Check sheet for the modelled part. Datum: model origin and axes. Units: mm. Round coordinates to 2 decimals unless told otherwise and drop trailing zeros. Order: outer loops, then holes, each group sorted by start corner. A loop starts at its lowest first (then second) coordinate and runs counter-clockwise, first axis right, second up. Notation, with made-up numbers: (-15.5, 37) -> (35.5, 37) arc R26 ccw to (35.5, 68) -> close; hole circle Ø1 at (63.25, 41). An arc over 180 degrees is marked (long way). Use CSV: the item, a comma, the result in double quotes.
```python
from build123d import *

# Parameters (mm, degrees)
SKETCH_1_R      = 1.5
EXTRUDE_1_DEPTH = 10


with BuildPart() as part:
    # 草图1 → 凸台-拉伸1 (new body)
    # profile 1 of 7: a face of its own
    with BuildSketch(Plane.XY):
        with BuildLine():
            Line((-33.5, 22.75), (-39.5, 22.75))
            Line((-39.5, 22.75), (-39.5, 9.98))
            Line((-39.5, 9.98), (-39.5, -22.75))
            Line((-39.5, -22.75), (-33.5, -22.75))
            Line((-33.5, -22.75), (39.5, -22.75))
            Line((39.5, -22.75), (39.5, 22.75))
            Line((39.5, 22.75), (6, 22.75))
            Line((6, 22.75), (6, 16.75))
            Line((6, 16.75), (3.578873161, 16.75))
            ThreePointArc((3.578873161, 16.75), (2.780687719, 16.52), (1.982502277, 16.75))
            Line((1.982502277, 16.75), (0, 16.75))
            Line((0, 16.75), (-1.982502277, 16.75))
            ThreePointArc((-1.982502277, 16.75), (-2.780687719, 16.52), (-3.578873161, 16.75))
            Line((-3.578873161, 16.75), (-6, 16.75))
            Line((-6, 16.75), (-6, 22.75))
            Line((-6, 22.75), (-33.5, 22.75))
        make_face()
        with Locations((-36.5, -17.48)):
            Circle(SKETCH_1_R, mode=Mode.SUBTRACT)
        with BuildLine():
            ThreePointArc((-29, -17.48), (-30.5, -18.98), (-32, -17.48))
            ThreePointArc((-32, -17.48), (-30.5, -15.98), (-29, -17.48))
        make_face(mode=Mode.SUBTRACT)
        with Locations((30.5, -17.48)):
            Circle(SKETCH_1_R, mode=Mode.SUBTRACT)
        with Locations((36.5, -17.48)):
            Circle(SKETCH_1_R, mode=Mode.SUBTRACT)
        with Locations((-36.5, 8.02)):
            Circle(SKETCH_1_R, mode=Mode.SUBTRACT)
        with BuildLine():
            ThreePointArc((-29, 8.02), (-30.5, 6.52), (-32, 8.02))
            ThreePointArc((-32, 8.02), (-30.5, 9.52), (-29, 8.02))
        make_face(mode=Mode.SUBTRACT)
        with Locations((-36.5, 18.02)):
            Circle(SKETCH_1_R, mode=Mode.SUBTRACT)
        with Locations((30.5, 8.02)):
            Circle(SKETCH_1_R, mode=Mode.SUBTRACT)
        with Locations((36.5, 8.02)):
            Circle(SKETCH_1_R, mode=Mode.SUBTRACT)
        with Locations((36.5, 18.02)):
            Circle(SKETCH_1_R, mode=Mode.SUBTRACT)
    # profile 2 of 7: a face of its own
    with BuildSketch(Plane.XY):
        with BuildLine():
            Line((-33.5, 22.75), (-39.5, 22.75))
            Line((-39.5, 22.75), (-39.5, 9.98))
            Line((-39.5, 9.98), (-39.5, -22.75))
            Line((-39.5, -22.75), (-33.5, -22.75))
            Line((-33.5, -22.75), (39.5, -22.75))
            Line((39.5, -22.75), (39.5, 22.75))
            Line((39.5, 22.75), (6, 22.75))
            Line((6, 22.75), (6, 16.75))
            Line((6, 16.75), (3.578873161, 16.75))
            ThreePointArc((3.578873161, 16.75), (2.780687719, 16.52), (1.982502277, 16.75))
            Line((1.982502277, 16.75), (0, 16.75))
            Line((0, 16.75), (-1.982502277, 16.75))
            ThreePointArc((-1.982502277, 16.75), (-2.780687719, 16.52), (-3.578873161, 16.75))
            Line((-3.578873161, 16.75), (-6, 16.75))
            Line((-6, 16.75), (-6, 22.75))
            Line((-6, 22.75), (-33.5, 22.75))
        make_face()
        with Locations((-36.5, -17.48)):
            Circle(SKETCH_1_R, mode=Mode.SUBTRACT)
        with BuildLine():
            ThreePointArc((-29, -17.48), (-30.5, -18.98), (-32, -17.48))
            ThreePointArc((-32, -17.48), (-30.5, -15.98), (-29, -17.48))
        make_face(mode=Mode.SUBTRACT)
        with Locations((30.5, -17.48)):
            Circle(SKETCH_1_R, mode=Mode.SUBTRACT)
        with Locations((36.5, -17.48)):
            Circle(SKETCH_1_R, mode=Mode.SUBTRACT)
        with Locations((-36.5, 8.02)):
            Circle(SKETCH_1_R, mode=Mode.SUBTRACT)
        with BuildLine():
            ThreePointArc((-29, 8.02), (-30.5, 6.52), (-32, 8.02))
            ThreePointArc((-32, 8.02), (-30.5, 9.52), (-29, 8.02))
        make_face(mode=Mode.SUBTRACT)
        with Locations((-36.5, 18.02)):
            Circle(SKETCH_1_R, mode=Mode.SUBTRACT)
        with Locations((30.5, 8.02)):
            Circle(SKETCH_1_R, mode=Mode.SUBTRACT)
        with Locations((36.5, 8.02)):
            Circle(SKETCH_1_R, mode=Mode.SUBTRACT)
        with Locations((36.5, 18.02)):
            Circle(SKETCH_1_R, mode=Mode.SUBTRACT)
    # profile 3 of 7: a face of its own
    with BuildSketch(Plane.XY):
        with BuildLine():
            Line((-33.5, 22.75), (-39.5, 22.75))
            Line((-39.5, 22.75), (-39.5, 9.98))
            Line((-39.5, 9.98), (-39.5, -22.75))
            Line((-39.5, -22.75), (-33.5, -22.75))
            Line((-33.5, -22.75), (39.5, -22.75))
            Line((39.5, -22.75), (39.5, 22.75))
            Line((39.5, 22.75), (6, 22.75))
            Line((6, 22.75), (6, 16.75))
            Line((6, 16.75), (3.578873161, 16.75))
            ThreePointArc((3.578873161, 16.75), (2.780687719, 16.52), (1.982502277, 16.75))
            Line((1.982502277, 16.75), (0, 16.75))
            Line((0, 16.75), (-1.982502277, 16.75))
            ThreePointArc((-1.982502277, 16.75), (-2.780687719, 16.52), (-3.578873161, 16.75))
            Line((-3.578873161, 16.75), (-6, 16.75))
            Line((-6, 16.75), (-6, 22.75))
            Line((-6, 22.75), (-33.5, 22.75))
        make_face()
        with Locations((-36.5, -17.48)):
            Circle(SKETCH_1_R, mode=Mode.SUBTRACT)
        with BuildLine():
            ThreePointArc((-29, -17.48), (-30.5, -18.98), (-32, -17.48))
            ThreePointArc((-32, -17.48), (-30.5, -15.98), (-29, -17.48))
        make_face(mode=Mode.SUBTRACT)
        with Locations((30.5, -17.48)):
            Circle(SKETCH_1_R, mode=Mode.SUBTRACT)
        with Locations((36.5, -17.48)):
            Circle(SKETCH_1_R, mode=Mode.SUBTRACT)
        with Locations((-36.5, 8.02)):
            Circle(SKETCH_1_R, mode=Mode.SUBTRACT)
        with BuildLine():
            ThreePointArc((-29, 8.02), (-30.5, 6.52), (-32, 8.02))
            ThreePointArc((-32, 8.02), (-30.5, 9.52), (-29, 8.02))
        make_face(mode=Mode.SUBTRACT)
        with Locations((-36.5, 18.02)):
            Circle(SKETCH_1_R, mode=Mode.SUBTRACT)
        with Locations((30.5, 8.02)):
            Circle(SKETCH_1_R, mode=Mode.SUBTRACT)
        with Locations((36.5, 8.02)):
            Circle(SKETCH_1_R, mode=Mode.SUBTRACT)
        with Locations((36.5, 18.02)):
            Circle(SKETCH_1_R, mode=Mode.SUBTRACT)
    # profile 4 of 7: a face of its own
    with BuildSketch(Plane.XY):
        with BuildLine():
            Line((0, 22.75), (-6, 22.75))
            Line((-6, 22.75), (-6, 16.75))
            Line((-6, 16.75), (-3.578873161, 16.75))
            ThreePointArc((-3.578873161, 16.75), (-3.506195071, 19.332874359), (-1.280687719, 18.02))
            ThreePointArc((-1.280687719, 18.02), (-1.46781336, 17.294492648), (-1.982502277, 16.75))
            Line((-1.982502277, 16.75), (0, 16.75))
            Line((0, 16.75), (0, 22.75))
        make_face()
    # profile 5 of 7: a face of its own
    with BuildSketch(Plane.XY):
        with BuildLine():
            Line((6, 22.75), (0, 22.75))
            Line((0, 22.75), (0, 16.75))
            Line((0, 16.75), (1.982502277, 16.75))
            ThreePointArc((1.982502277, 16.75), (2.055180366, 19.332874359), (4.280687719, 18.02))
            ThreePointArc((4.280687719, 18.02), (4.093562078, 17.294492648), (3.578873161, 16.75))
            Line((3.578873161, 16.75), (6, 16.75))
            Line((6, 16.75), (6, 22.75))
        make_face()
    # profile 6 of 7: a face of its own
    with BuildSketch(Plane.XY):
        with BuildLine():
            Line((-33.5, 22.75), (-39.5, 22.75))
            Line((-39.5, 22.75), (-39.5, 9.98))
            Line((-39.5, 9.98), (-39.5, -22.75))
            Line((-39.5, -22.75), (-33.5, -22.75))
            Line((-33.5, -22.75), (39.5, -22.75))
            Line((39.5, -22.75), (39.5, 22.75))
            Line((39.5, 22.75), (6, 22.75))
            Line((6, 22.75), (6, 16.75))
            Line((6, 16.75), (3.578873161, 16.75))
            ThreePointArc((3.578873161, 16.75), (2.780687719, 16.52), (1.982502277, 16.75))
            Line((1.982502277, 16.75), (0, 16.75))
            Line((0, 16.75), (-1.982502277, 16.75))
            ThreePointArc((-1.982502277, 16.75), (-2.780687719, 16.52), (-3.578873161, 16.75))
            Line((-3.578873161, 16.75), (-6, 16.75))
            Line((-6, 16.75), (-6, 22.75))
            Line((-6, 22.75), (-33.5, 22.75))
        make_face()
        with Locations((-36.5, -17.48)):
            Circle(SKETCH_1_R, mode=Mode.SUBTRACT)
        with BuildLine():
            ThreePointArc((-29, -17.48), (-30.5, -18.98), (-32, -17.48))
            ThreePointArc((-32, -17.48), (-30.5, -15.98), (-29, -17.48))
        make_face(mode=Mode.SUBTRACT)
        with Locations((30.5, -17.48)):
            Circle(SKETCH_1_R, mode=Mode.SUBTRACT)
        with Locations((36.5, -17.48)):
            Circle(SKETCH_1_R, mode=Mode.SUBTRACT)
        with Locations((-36.5, 8.02)):
            Circle(SKETCH_1_R, mode=Mode.SUBTRACT)
        with BuildLine():
            ThreePointArc((-29, 8.02), (-30.5, 6.52), (-32, 8.02))
            ThreePointArc((-32, 8.02), (-30.5, 9.52), (-29, 8.02))
        make_face(mode=Mode.SUBTRACT)
        with Locations((-36.5, 18.02)):
            Circle(SKETCH_1_R, mode=Mode.SUBTRACT)
        with Locations((30.5, 8.02)):
            Circle(SKETCH_1_R, mode=Mode.SUBTRACT)
        with Locations((36.5, 8.02)):
            Circle(SKETCH_1_R, mode=Mode.SUBTRACT)
        with Locations((36.5, 18.02)):
            Circle(SKETCH_1_R, mode=Mode.SUBTRACT)
    # profile 7 of 7: a face of its own
    with BuildSketch(Plane.XY):
        with BuildLine():
            Line((-33.5, 22.75), (-39.5, 22.75))
            Line((-39.5, 22.75), (-39.5, 9.98))
            Line((-39.5, 9.98), (-39.5, -22.75))
            Line((-39.5, -22.75), (-33.5, -22.75))
            Line((-33.5, -22.75), (39.5, -22.75))
            Line((39.5, -22.75), (39.5, 22.75))
            Line((39.5, 22.75), (6, 22.75))
            Line((6, 22.75), (6, 16.75))
            Line((6, 16.75), (3.578873161, 16.75))
            ThreePointArc((3.578873161, 16.75), (2.780687719, 16.52), (1.982502277, 16.75))
            Line((1.982502277, 16.75), (0, 16.75))
            Line((0, 16.75), (-1.982502277, 16.75))
            ThreePointArc((-1.982502277, 16.75), (-2.780687719, 16.52), (-3.578873161, 16.75))
            Line((-3.578873161, 16.75), (-6, 16.75))
            Line((-6, 16.75), (-6, 22.75))
            Line((-6, 22.75), (-33.5, 22.75))
        make_face()
        with Locations((-36.5, -17.48)):
            Circle(SKETCH_1_R, mode=Mode.SUBTRACT)
        with BuildLine():
            ThreePointArc((-29, -17.48), (-30.5, -18.98), (-32, -17.48))
            ThreePointArc((-32, -17.48), (-30.5, -15.98), (-29, -17.48))
        make_face(mode=Mode.SUBTRACT)
        with Locations((30.5, -17.48)):
            Circle(SKETCH_1_R, mode=Mode.SUBTRACT)
        with Locations((36.5, -17.48)):
            Circle(SKETCH_1_R, mode=Mode.SUBTRACT)
        with Locations((-36.5, 8.02)):
            Circle(SKETCH_1_R, mode=Mode.SUBTRACT)
        with BuildLine():
            ThreePointArc((-29, 8.02), (-30.5, 6.52), (-32, 8.02))
            ThreePointArc((-32, 8.02), (-30.5, 9.52), (-29, 8.02))
        make_face(mode=Mode.SUBTRACT)
        with Locations((-36.5, 18.02)):
            Circle(SKETCH_1_R, mode=Mode.SUBTRACT)
        with Locations((30.5, 8.02)):
            Circle(SKETCH_1_R, mode=Mode.SUBTRACT)
        with Locations((36.5, 8.02)):
            Circle(SKETCH_1_R, mode=Mode.SUBTRACT)
        with Locations((36.5, 18.02)):
            Circle(SKETCH_1_R, mode=Mode.SUBTRACT)
    extrude(amount=EXTRUDE_1_DEPTH)


solid = part.part
```
Q1. Sectioned sample at D-D, the plane z = 8.5. State how many separate pieces and enclosed holes the cut face has, then the cut area to 3 significant figures.
Result sheet:
separate pieces,"1"
enclosed holes,"12"
area,"3,510 mm^2"
Q2. Sectioned sample at B-B, the plane x = 30.5. Enter the section's corners in (y, z), then the cut area to 3 significant figures.
Result sheet:
outline,"(-22.75, 0) -> (-18.98, 0) -> (-18.98, 10) -> (-22.75, 10) -> close; (-15.98, 0) -> (6.52, 0) -> (6.52, 10) -> (-15.98, 10) -> close; (9.52, 0) -> (22.75, 0) -> (22.75, 10) -> (9.52, 10) -> close"
area,"395 mm^2"
Q3. Sectioned sample at C-C, the plane x = -36.5. Enter the section's corners in (y, z).
Result sheet:
outline,"(-22.75, 0) -> (-18.98, 0) -> (-18.98, 10) -> (-22.75, 10) -> close; (-15.98, 0) -> (6.52, 0) -> (6.52, 10) -> (-15.98, 10) -> close; (9.52, 0) -> (16.52, 0) -> (16.52, 10) -> (9.52, 10) -> close; (19.52, 0) -> (22.75, 0) -> (22.75, 10) -> (19.52, 10) -> close"
Q4. Go/stop test with a flat-tipped pin: pin 1 (4 mm diameter, centred on x = -30.5, y = -17.48, fed in from +Z). Record where the tip stops, or that it passes through.
Result sheet:
pin 1,"stops at z = 10"
Q5. Mould release check, pull along X, two halves, no side actions. Record for faces 1 (the face through (29, 8, 5)), 2 (the face through (-39.5, 0, 5)), 3 (the face through (1, 22.75, 5)): pulls with the +X half, pulls with the -X half, needs draft (parallel to the pull), parting line crosses it, or undercut.
Result sheet:
face 1,"undercut"
face 2,"pulls with the -X half"
face 3,"needs draft"
Q6. Sectioned sample at A-A, the plane y = 8.02. Enter the section's corners in (x, z).
Result sheet:
outline,"(-39.5, 0) -> (-38, 0) -> (-38, 10) -> (-39.5, 10) -> close; (-35, 0) -> (-32, 0) -> (-32, 10) -> (-35, 10) -> close; (-29, 0) -> (29, 0) -> (29, 10) -> (-29, 10) -> close; (32, 0) -> (35, 0) -> (35, 10) -> (32, 10) -> close; (38, 0) -> (39.5, 0) -> (39.5, 10) -> (38, 10) -> close"
Q7. Scan lines: L1, parallel to Y at x = -36.5, z = 2.25; L2, parallel to Y at x = 30.5, z = 6; L3, parallel to X at y = -17, z = 9.25. Record each from-to range of solid material in increasing order.
Result sheet:
L1,"y = -22.75 to -18.98, -15.98 to 6.52, 9.52 to 16.52, 19.52 to 22.75"
L2,"y = -22.75 to -18.98, -15.98 to 6.52, 9.52 to 22.75"
L3,"x = -39.5 to -37.92, -35.08 to -31.92, -29.08 to 29.08, 31.92 to 35.08, 37.92 to 39.5"
